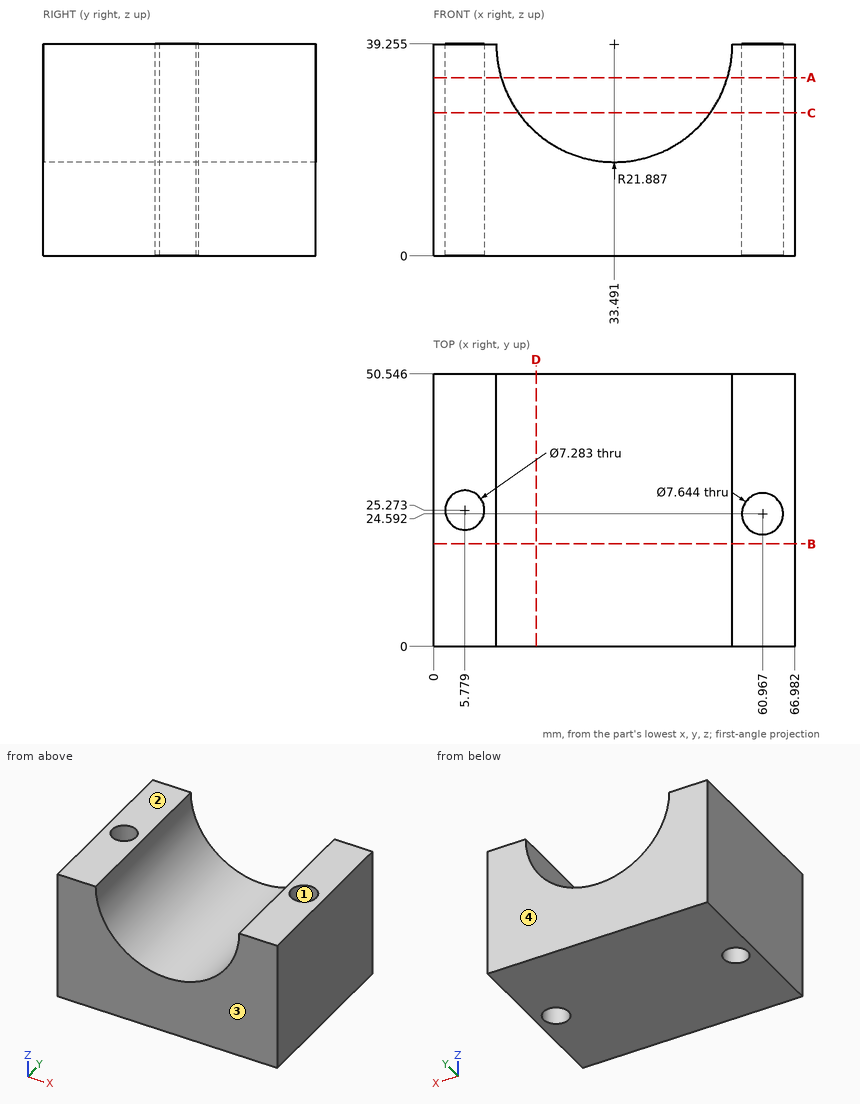
Source: three-view drawing plus pictorial views. Frame: mm from the lowest corner of the part. Give positions to 0.01 mm unless a question says otherwise; leave off trailing zeros. Loops run counter-clockwise (first coordinate to the right, second up) from the corner with the lowest first, then second, coordinate; pieces in that order, holes last. Notation, with made-up numbers: (-30, 44.25) -> (26, 44.25) arc R16 cw to (26, 70.25) -> close; hole circle Ø5 at (84.5, 45.25). An arc over 180 degrees is marked (long way). Put each result on its own line as item: value. Start each with the question number.
1) Cut plane A-A (z = 33). Return loops of the section in (x, y) (1 decimal), then the cut area to 3 significant figures.
2) Draft query along Y for the marked faces 1, 2, 3 and 4. Return one class per face: released by +Y, released by -Y, zero draft, split by the parting line, or undercut.
3) Cut plane B-B (y = 19). Return loops of the section in (x, z) (1 decimal), then the cut area to 3 significant figures.
4) Material intervals for probe 1 along Z at (x, y) = (52.5, 40.5) (1 decimal); probe 2 along Y at (x, z) = (4.5, 4.5) (1 decimal); probe 3 along X at (y, z) = (27, 29) (1 decimal), sorted ascending.
5) Cut plane C-C (z = 26.5). Return loops of the section in (x, y) (1 decimal).
6) Cut plane D-D (x = 19). Return loops of the section in (y, z), then the cut area to 4 significant figures.
Results are:
1. outline: (0, 0) -> (12.5, 0) -> (12.5, 50.5) -> (0, 50.5) -> close; (54.5, 0) -> (67, 0) -> (67, 50.5) -> (54.5, 50.5) -> close; hole circle Ø7.3 at (5.8, 25.3); hole circle Ø7.6 at (61, 24.6)
1. area: 1,180 mm2
2. face 1: undercut
2. face 2: zero draft
2. face 3: released by -Y
2. face 4: released by +Y
3. outline: (0, 0) -> (67, 0) -> (67, 39.3) -> (55.4, 39.3) arc R21.9 cw to (11.6, 39.3) -> (0, 39.3) -> close
3. area: 1,880 mm2
4. probe 1: z = 0 to 28.4
4. probe 2: y = 0 to 21.9, 28.7 to 50.5
4. probe 3: x = 0 to 2.6, 9 to 14.2, 52.8 to 58, 63.9 to 67
5. outline: (0, 0) -> (15.7, 0) -> (15.7, 50.5) -> (0, 50.5) -> close; (51.3, 0) -> (67, 0) -> (67, 50.5) -> (51.3, 50.5) -> close; hole circle Ø7.3 at (5.8, 25.3); hole circle Ø7.6 at (61, 24.6)
6. outline: (0, 0) -> (50.55, 0) -> (50.55, 22.85) -> (0, 22.85) -> close
6. area: 1,155 mm2
